Source: CAD feature listing. Evaluate the final solid. Frame: model axes, mm. Face numbers are marked on the shaded views. A direction names the side the tool comes from. Round coordinates to 2 decimals unless told otherwise and drop trailing zeros. Loops run counter-clockwise (first coordinate to the right, second up) from the corner with the lowest first, then second, coordinate; pieces in that order, holes last. Notation, with made-up numbers: M 58.25,85 L 106.25,85 A4 cw 106.25,90 Z; hole C 10,72.25 d2. An arc over 180 degrees is marked long. Answer as a JSON object with one key per item and string values.
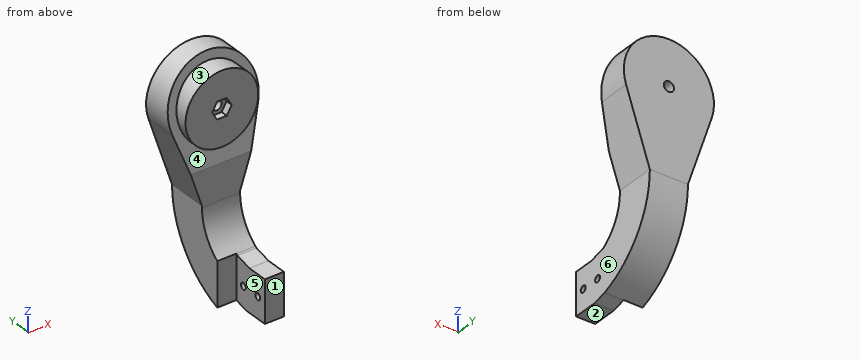
from build123d import *

# Parameters (mm, degrees)
CROQUIS1_R              = 21
SALIENTE_EXTRUIR1_DEPTH = 24
CROQUIS2_R              = 2.9
CORTAR_EXTRUIR1_DEPTH   = 30
CROQUIS3_R              = 26
SALIENTE_EXTRUIR2_DEPTH = 12
SALIENTE_EXTRUIR3_DEPTH = 26
CROQUIS6_W              = 19.429
CROQUIS6_H              = 23.308672713
SALIENTE_EXTRUIR4_DEPTH = 52
CORTAR_EXTRUIR2_DEPTH   = 61.862693955
SALIENTE_EXTRUIR5_DEPTH = 11
SALIENTE_EXTRUIR6_DEPTH = 11
CROQUIS10_R             = 1.9
CORTAR_EXTRUIR3_DEPTH   = 110.615590995
CROQUIS11_R             = 2.9
CORTAR_EXTRUIR4_DEPTH   = 120.153595066
CORTAR_EXTRUIR5_DEPTH   = 4


with BuildPart() as part:
    # Croquis1 → Saliente-Extruir1 (new body)
    with BuildSketch(Plane(origin=(0, 0, 0), x_dir=(1, 0, 0), z_dir=(0, 1, 0))):
        with Locations(Location((0, 0, 0), (0, 0, 270))):
            Circle(CROQUIS1_R)
    extrude(amount=SALIENTE_EXTRUIR1_DEPTH)

    # Croquis2 → Cortar-Extruir1 (cut, symmetric)
    with BuildSketch(Plane(origin=(0, 24, 0), x_dir=(1, 0, 0), z_dir=(0, 1, 0))):
        with Locations(Location((0, 0, 0), (0, 0, 270))):
            Circle(CROQUIS2_R)
    extrude(amount=CORTAR_EXTRUIR1_DEPTH, both=True, mode=Mode.SUBTRACT)

    # Croquis3 → Saliente-Extruir2 (add)
    with BuildSketch(Plane(origin=(0, 24, 0), x_dir=(1, 0, 0), z_dir=(0, 1, 0))):
        with Locations(Location((0, 0, 0), (0, 0, 270))):
            Circle(CROQUIS3_R)
    extrude(amount=-SALIENTE_EXTRUIR2_DEPTH)

    # Croquis4 → Saliente-Extruir3 (add, symmetric)
    with BuildSketch(Plane(origin=(0, 0, 0), x_dir=(0, 0, -1), z_dir=(1, 0, 0))):
        Polygon((-26, 13.930297777), (-26, 12), (30.091374751, 0.691327287), (30.091374751, 24), (-26, 24), align=None)
    extrude(amount=SALIENTE_EXTRUIR3_DEPTH, both=True)

    # Croquis6 → Saliente-Extruir4 (add)
    with BuildSketch(Plane(origin=(26, 0, 0), x_dir=(0, 0, -1), z_dir=(1, 0, 0))):
        with Locations((39.805874751, 12.345663644)):
            Rectangle(CROQUIS6_W, CROQUIS6_H)
    extrude(amount=-SALIENTE_EXTRUIR4_DEPTH)

    # Croquis5 → Cortar-Extruir2 (cut, through all)
    with BuildSketch(Plane(origin=(0, 24, 0), x_dir=(1, 0, 0), z_dir=(0, 1, 0))):
        with BuildLine():
            Line((-31.296292427, 177.340731999), (24.68369475, 8.167938142))
            ThreePointArc((24.68369475, 8.167938142), (0, -26), (-24.68369475, 8.167938142))
            Line((-24.68369475, 8.167938142), (-11, 49.520374751))
            Line((-11, 49.520374751), (11, 49.520374751))
            Line((11, 49.520374751), (24.68369475, 8.167938142))
            Line((24.68369475, 8.167938142), (26, 49.520374751))
            Line((26, 49.520374751), (11, 49.520374751))
            Line((11, 49.520374751), (-167.194256769, 49.520374751))
            Line((-167.194256769, 49.520374751), (76.977143024, -210.081435923))
            Line((76.977143024, -210.081435923), (212.875107366, -82.261078675))
            Line((212.875107366, -82.261078675), (-31.296292427, 177.340731999))
        make_face()
    extrude(amount=-CORTAR_EXTRUIR2_DEPTH, mode=Mode.SUBTRACT)


with BuildPart() as cortar_extruir2_kept_piece:
    # of the separate pieces the step leaves, the one the design keeps (cortar_extruir2_pieces_kept)
    add(part.part.solids().sort_by_distance((0, 0, 21))[0])

    # Croquis7 → Saliente-Extruir5 (add, symmetric)
    with BuildSketch(Plane(origin=(0, 0, 0), x_dir=(0, 0, -1), z_dir=(1, 0, 0))):
        with BuildLine():
            Line((49.520374751, 24), (49.520374751, 0.691327287))
            Line((49.520374751, 0.691327287), (50.478144868, 0.691327287))
            ThreePointArc((50.478144868, 0.691327287), (63.55673371, -2.469267031), (73.748722442, -11.253469229))
            Line((73.748722442, -11.253469229), (99.248722442, -11.253469229))
            ThreePointArc((99.248722442, -11.253469229), (79.998709912, 14.292570123), (49.520374751, 24))
        make_face()
    extrude(amount=SALIENTE_EXTRUIR5_DEPTH, both=True)

    # Croquis9 → Saliente-Extruir6 (add)
    with BuildSketch(Plane(origin=(11, 0, 0), x_dir=(0, 0, -1), z_dir=(1, 0, 0))):
        with BuildLine():
            Line((101.09458803, -18.883363084), (99.248722442, -11.253469229))
            Line((99.248722442, -11.253469229), (73.748722442, -11.253469229))
            ThreePointArc((73.748722483, -11.2534692), (74.042597019, -11.670890415), (74.32898512, -12.093483089))
            ThreePointArc((74.32898512, -12.093483089), (77.894859555, -19.667595219), (79.118326526, -27.949247445))
            ThreePointArc((79.118326526, -27.949247445), (78.984304271, -30.716755499), (78.583491791, -33.458363084))
            Line((78.583491791, -33.458363084), (101.09458803, -33.458363084))
            Line((101.09458803, -33.458363084), (101.09458803, -18.883363084))
        make_face()
        with BuildLine():
            ThreePointArc((79.118326526, -27.949247445), (77.894859555, -19.667595219), (74.32898512, -12.093483089))
            Line((74.32898512, -12.093483089), (76.59458803, -21.458363084))
            Line((76.59458803, -21.458363084), (76.59458803, -33.458363084))
            Line((76.59458803, -33.458363084), (78.583491791, -33.458363084))
            ThreePointArc((78.583491791, -33.458363084), (78.984304271, -30.716755499), (79.118326526, -27.949247445))
        make_face()
    extrude(amount=-SALIENTE_EXTRUIR6_DEPTH)

    # Croquis10 → Cortar-Extruir3 (cut, through all)
    with BuildSketch(Plane.ZY):
        with Locations((-88.84458803, -27.958363084)):
            Circle(CROQUIS10_R)
        with Locations((-88.84458803, -16.728363084)):
            Circle(CROQUIS10_R)
    extrude(amount=-CORTAR_EXTRUIR3_DEPTH, mode=Mode.SUBTRACT)

    # Croquis11 → Cortar-Extruir4 (cut, through all)
    with BuildSketch(Plane(origin=(0, 24, 0), x_dir=(1, 0, 0), z_dir=(0, 1, 0))):
        with Locations(Location((0, 0, 0), (0, 0, 270))):
            Circle(CROQUIS11_R)
    extrude(amount=-CORTAR_EXTRUIR4_DEPTH, mode=Mode.SUBTRACT)

    # Croquis12 → Cortar-Extruir5 (cut)
    with BuildSketch(Plane.XZ):
        Polygon((2.825, 4.893043531), (-2.825, 4.893043531), (-5.65, 0), (-2.825, -4.893043531), (2.825, -4.893043531), (5.65, 0), align=None)
    extrude(amount=-CORTAR_EXTRUIR5_DEPTH, mode=Mode.SUBTRACT)


solid = cortar_extruir2_kept_piece.part
Item 1: Contact query for flat-ended pins moving along their axis: pin 1 Ø3 at (x, y) = (1, 2) entering from +Z; pin 2 Ø16.5 at (x, z) = (-2, -41.5) entering from -Y; pin 3 Ø18 at (y, z) = (-20.5, -87) entering from -X; pin 4 Ø3 at (y, z) = (-27.96, -88.84) entering from -X. Output: stop coordinate, or through.
Answer sheet:
{"pin 1": "stops at z = 21", "pin 2": "stops at y = 0.69", "pin 3": "stops at x = 0", "pin 4": "passes through"}
Item 2: Pull-direction query (Z, two-part tool) for the marked faces 1, 2 and 3; classes: pulls with the +Z half, pulls with the -Z half, needs draft (parallel to the pull), parting line crosses it, or undercut.
Answer sheet:
{"face 1": "needs draft", "face 2": "pulls with the -Z half", "face 3": "undercut"}
Item 3: Section C-C on y = -9.5. Return the cut outline in (x, z), then the cut area to 3 significant figures.
Answer sheet:
{"outline": "M -11,-98.6 L 11,-98.6 L 11,-72.38 L -11,-72.38 Z", "area": "577 mm²"}
Item 4: Line query: probe 1 along X at (y, z) = (12, 0); probe 2 along X at (y, z) = (17.5, -1); probe 3 along Y at (x, z) = (-15.5, 1). Output: solid intervals per line, ascending. Write a range as from..to.
Answer sheet:
{"probe 1": "x = -26..-2.9, 2.9..26", "probe 2": "x = -25.98..-2.72, 2.72..25.98", "probe 3": "y = 0..24"}
Item 5: Access query for the marked faces 4, 5 and 6. Directions: +Z, -Z, +X, -X, +Y, -Y. A direction counts if a zero-diameter tool reaches every point of the face in a straight line with its end or side. Return the directions, or none.
Answer sheet:
{"face 4": "-Y", "face 5": "+Z, -Z, -X, -Y", "face 6": "-Z, +X, +Y, -Y"}
Item 6: Section A-A on y = 20. Return the cut outline in (x, z), then the cut area to 3 significant figures.
Answer sheet:
{"outline": "M -24.68,-8.17 L -11,-49.52 L -11,-69.66 L 11,-69.66 L 11,-49.52 L 24.68,-8.17 A26 ccw long Z; hole C 0,0 d5.8", "area": "3,370 mm²"}
Item 7: Section B-B on z = -80.5. Return the cut outline in (x, y), then the cut area to 3 significant figures.
Answer sheet:
{"outline": "M -11,-11.25 L 0,-11.25 L 0,-33.46 L 11,-33.46 L 11,13.93 L -11,13.93 Z", "area": "798 mm²"}
Item 8: Section D-D on z = -35. Return the cut outline in (x, y), then the cut area to 3 significant figures.
Answer sheet:
{"outline": "M -15.8,0.69 L 15.8,0.69 L 15.8,24 L -15.8,24 Z", "area": "737 mm²"}
